from build123d import *

# Parameters (mm, degrees)
F0_R      = 11
F1_DEPTH  = 40
F3_SIZE   = 2
F4_SIZE   = 2
F5_R      = 19.577799
F6_DEPTH  = 8
F8_R      = 6
F9_DEPTH  = 30
F11_R     = 4
F12_DEPTH = 33.578799
F15_DEPTH = 10.578799
F17_DEPTH = 25


with BuildPart() as f1:
    # F0 (on Top) → F1 (new body, symmetric)
    with BuildSketch(Plane.XY):
        Circle(F0_R)
    extrude(amount=F1_DEPTH, both=True)

    # F3
    f3_edges = [f1.edges().sort_by_distance(p)[0] for p in [
        (-11, 0, 40),
    ]]
    chamfer(f3_edges, length=F3_SIZE)

    # F4
    f4_edges = [f1.edges().sort_by_distance(p)[0] for p in [
        (-11, 0, -40),
    ]]
    chamfer(f4_edges, length=F4_SIZE)

    # F5 (on Top) → F6 (join, symmetric)
    with BuildSketch(Plane.XY):
        Circle(F5_R)
    extrude(amount=F6_DEPTH, both=True)

    # F8 (on offset) → F9 (cut)
    with BuildSketch(Plane.YZ.offset(14)):
        Circle(F8_R)
    extrude(amount=F9_DEPTH, mode=Mode.SUBTRACT)

    # F11 (on offset) → F12 (cut, through all)
    with BuildSketch(Plane.YZ.offset(14)):
        Circle(F11_R)
    extrude(amount=-F12_DEPTH, mode=Mode.SUBTRACT)

    # F14 (on offset) → F15 (cut, through all)
    with BuildSketch(Plane.YZ.offset(9)):
        with BuildLine():
            Line((3, 18), (3, 30))
            ThreePointArc((3, 30), (0, 33), (-3, 30))
            Line((-3, 30), (-3, 18))
            ThreePointArc((-3, 18), (0, 15), (3, 18))
        make_face()
    extrude(amount=F15_DEPTH, mode=Mode.SUBTRACT)

    # F16 (on offset) → F17 (cut)
    with BuildSketch(Plane.YZ.offset(9)):
        with BuildLine():
            Line((-3, -18), (-3, -30))
            ThreePointArc((-3, -30), (0, -33), (3, -30))
            Line((3, -30), (3, -18))
            ThreePointArc((3, -18), (0, -15), (-3, -18))
        make_face()
    extrude(amount=F17_DEPTH, mode=Mode.SUBTRACT)


solid = f1.part
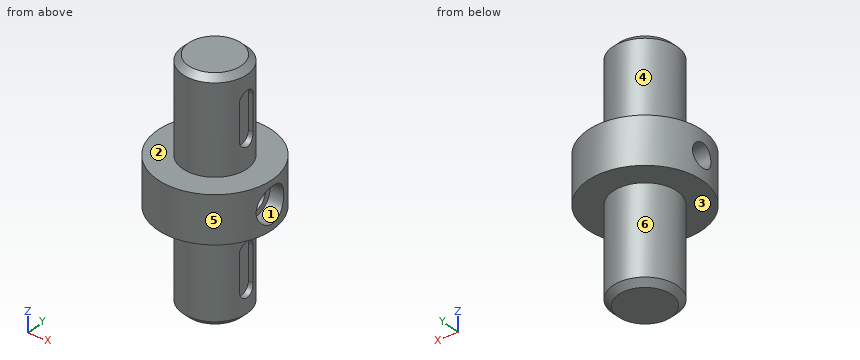
Could you check a few things on this model? Use its own coordinates, in mm. Face numbers are marked on the shaded views. A direction names the side the tool comes from. Give positions to 0.01 mm unless a question says otherwise; leave off trailing zeros. Order: outer loops, then holes, each group sorted by start corner. A loop starts at its lowest first (then second) coordinate and runs counter-clockwise, first axis right, second up.
Item 1: If we section it at C-C, the plane z = 26: Write out the boundary of the cut face in (x, y).
Item 2: I need wall thicknesses on line 1 (Y direction, x = 0, z = 0); line 2 (Z direction, x = 4.5, y = 0); line 3 (Z direction, x = 16.75, y = 0). Which ranges of each line are inside material? Lowest first, please.
Item 3: If we mould it in two halves opening along Z, with no side actions, what happens to the marked faces 1, 2 and 3? For each: pulls with the +Z half, pulls with the -Z half, needs draft (parallel to the pull), parting line crosses it, or undercut.
Item 4: If we section it at A-A, the plane x = 0: Write out the boundary of the cut face in (y, z).
Item 5: If we section it at D-D, the plane x = -13: Write out the boundary of the cut face in (y, z), plus the area to 3 significant figures.
Item 6: For the marked faces 4, 5 and 6, which set-ups out of +Z, -Z, +X, -X, +Y, -Y let a thin tool reach every point of the face, with its end or its side?
Item 7: I'm going to push flat-ended pins straight in: pin 1 (1.3 mm diameter, centred on x = 10, z = -26.5, fed in from +Y); pin 2 (1.3 mm diameter, centred on x = 9.5, z = 26.5, fed in from +Y); pin 3 (1 mm diameter, centred on x = -8, y = 14, fed in from +Z). Where does each tip first touch, or does it pass through?
Values:
1. outline: (9, -3) - (9, 3) - (10.58, 3) arc R11 ccw (long way) to (10.58, -3) - close
2. line 1: y = -19.58 to -4, 4 to 19.58
2. line 2: z = -40 to -4, 4 to 40
2. line 3: z = -8 to -6, 6 to 8
3. face 1: undercut
3. face 2: pulls with the +Z half
3. face 3: pulls with the -Z half
4. outline: (-19.58, -8) - (-11, -8) - (-11, -38) - (-9, -40) - (9, -40) - (11, -38) - (11, -8) - (19.58, -8) - (19.58, 8) - (11, 8) - (11, 38) - (9, 40) - (-9, 40) - (-11, 38) - (-11, 8) - (-19.58, 8) - close; hole circle Ø8 at (0, 0)
5. outline: (-14.64, -8) - (14.64, -8) - (14.64, 8) - (-14.64, 8) - close; hole circle Ø8 at (0, 0)
5. area: 418 mm2
6. face 4: +Z
6. face 5: +Z, -Z
6. face 6: -Z
7. pin 1: stops at y = 5.79
7. pin 2: stops at y = 6.53
7. pin 3: stops at z = 8
